Check sheet for the drawn part. Datum: minimum x, y, z corner. Units: mm. A direction names the side the tool comes from. Round coordinates to 2 decimals unless told otherwise and drop trailing zeros. Order: outer loops, then holes, each group sorted by start corner. A loop starts at its lowest first (then second) coordinate and runs counter-clockwise, first axis right, second up. Notation, with made-up numbers: (80.25, -13.5) -> (100.25, -13.5) arc R36 cw to (100.25, 23.5) -> close; hole circle Ø3 at (5, 5). An arc over 180 degrees is marked (long way). Use CSV: the item, a comma, the result in double quotes.
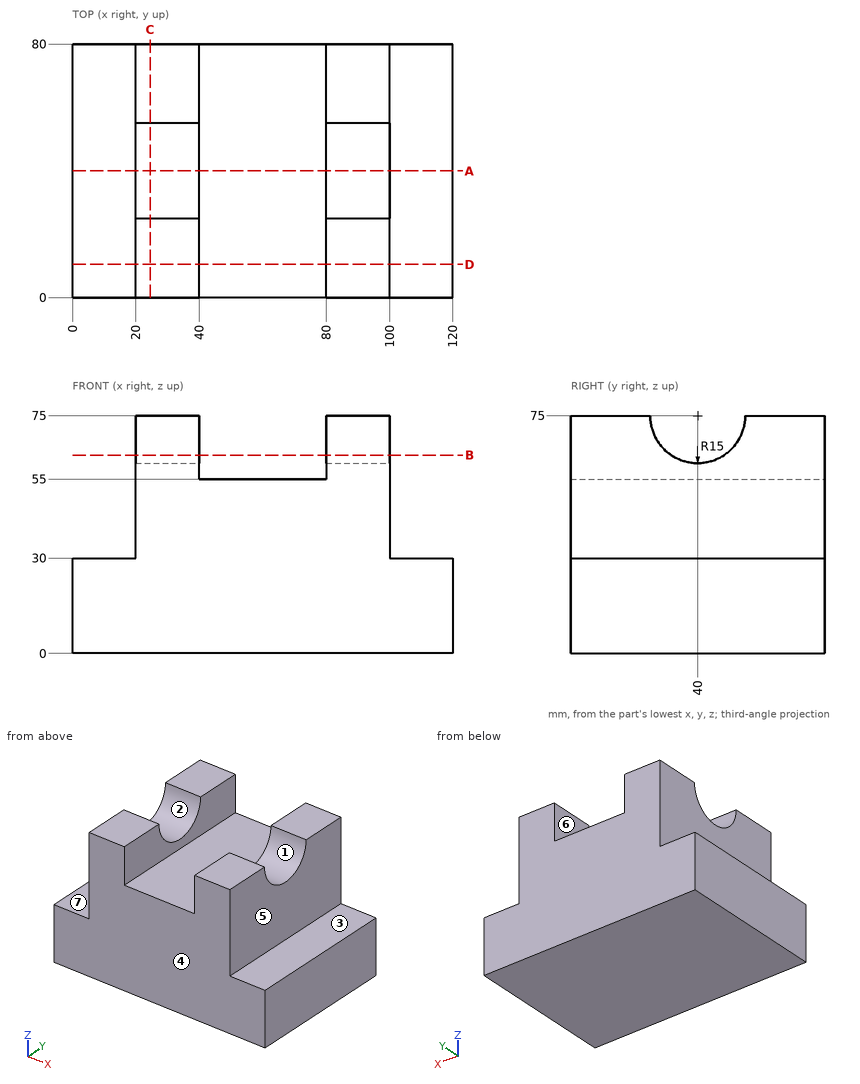
Q1. Sectioned sample at B-B, the plane z = 62.5. Enter the section's corners in (x, y).
Result sheet:
outline,"(20, 0) -> (40, 0) -> (40, 31.71) -> (20, 31.71) -> close; (20, 48.29) -> (40, 48.29) -> (40, 80) -> (20, 80) -> close; (80, 0) -> (100, 0) -> (100, 31.71) -> (80, 31.71) -> close; (80, 48.29) -> (100, 48.29) -> (100, 80) -> (80, 80) -> close"
Q2. Sectioned sample at C-C, the plane x = 24.5. Enter the section's corners in (y, z).
Result sheet:
outline,"(0, 0) -> (80, 0) -> (80, 75) -> (55, 75) arc R15 cw to (25, 75) -> (0, 75) -> close"
Q3. Scan lines: L1, parallel to X at y = 65, z = 67.5; L2, parallel to X at y = 13, z = 34; L3, parallel to Z at x = 113, y = 61. Record each from-to range of solid material in increasing order.
Result sheet:
L1,"x = 20 to 40, 80 to 100"
L2,"x = 20 to 100"
L3,"z = 0 to 30"
Q4. Sectioned sample at A-A, the plane y = 40. Enter the section's corners in (x, z), then the cut area to 3 significant figures.
Result sheet:
outline,"(0, 0) -> (120, 0) -> (120, 30) -> (100, 30) -> (100, 60) -> (80, 60) -> (80, 55) -> (40, 55) -> (40, 60) -> (20, 60) -> (20, 30) -> (0, 30) -> close"
area,"5,800 mm^2"
Q5. Go/stop test with flat-tipped pins: pin 1 (6 mm diameter, centred on x = 8.5, y = 32.5, fed in from +Z); pin 2 (12 mm diameter, centred on y = 68, z = 58.5, fed in from +X); pin 3 (3 mm diameter, centred on y = 23.5, z = 13.5, fed in from -X); pin 4 (2 mm diameter, centred on y = 42.5, z = 54, fed in from -X). Record where each tip stops, or that it passes through.
Result sheet:
pin 1,"stops at z = 30"
pin 2,"stops at x = 100"
pin 3,"stops at x = 0"
pin 4,"stops at x = 20"
Q6. Access from +Z, -Z, +X, -X, +Y, -Y to the whole of each face (thin tool, end or side, straight path). Record for the marked faces 5, 6 and 7.
Result sheet:
face 5,"+Z, +X, +Y, -Y"
face 6,"+Z, +Y, -Y"
face 7,"+Z, -X, +Y, -Y"
Q7. Sectioned sample at D-D, the plane y = 10.5. Enter the section's corners in (x, z).
Result sheet:
outline,"(0, 0) -> (120, 0) -> (120, 30) -> (100, 30) -> (100, 75) -> (80, 75) -> (80, 55) -> (40, 55) -> (40, 75) -> (20, 75) -> (20, 30) -> (0, 30) -> close"
Q8. Mould release check, pull along Y, two halves, no side actions. Record for the marked faces 1, 2, 3 and 4: pulls with the +Y half, pulls with the -Y half, needs draft (parallel to the pull), parting line crosses it, or undercut.
Result sheet:
face 1,"undercut"
face 2,"undercut"
face 3,"needs draft"
face 4,"pulls with the -Y half"
